Geometry check sheet. Reference: the model listing, model coordinates, mm. A direction names the side the tool comes from. Coordinates: 2 decimals unless noted, no trailing zeros. Order: outer loops, then holes, each group sorted by start corner. A loop starts at its lowest first (then second) coordinate and runs counter-clockwise, first axis right, second up. Notation, with made-up numbers: M 9.25,49.5 L 49.25,49.5 A8 ccw 49.25,58.5 Z; hole C 50.25,87.25 d8. An arc over 180 degrees is marked long. One line per item, written item: value. Start each with the question number.
1) Draft check along Z on faces 5 (the flat face through (-23, 0, 10)), 6 (the flat face through (22.47, 37.89, 16.47)), 7 (the flat face through (21.933, 37.891, 13.222)), 8 (the cylindrical face through (-0.323, -13.902, -15.247)). Enter one of: pulls with the +Z half, pulls with the -Z half, needs draft (parallel to the pull), parting line crosses it, or undercut.
2) Sectioned sample at B-B, the plane x = 0. Enter the section's corners in (y, z).
3) Sectioned sample at D-D, the plane y = 29.5. Enter the section's corners in (x, z), then the cut area to 3 significant figures.
4) Thickness scan on L1, parallel to X at y = 32.5, z = 0; L2, parallel to Y at x = -13.5, z = 24.5; L3, parallel to Y at x = -13, z = -30. Record the ranges inside material, lowest first. Write a range as from..to.
5) Go/stop test with flat-tipped pins: P1, Ø2, axis at x = 6.5, y = 30, coming from the -Z side; P2, Ø1.5, axis at y = 9.5, z = -1, coming from the -X side; P3, Ø3, axis at x = 25, y = 24.5, coming from the -Z side; P4, Ø1, axis at y = -13.5, z = 17, coming from the -X side. Record where each tip stops, or that it passes through.
6) Sectioned sample at A-A, the plane y = 37. Enter the section's corners in (x, z).
7) Access from +Z, -Z, +X, -X, +Y, -Y to the whole of each face (thin tool, end or side, straight path). Record for faces 1 (the flat face through (-23.08, 37.891, 15.624)), 2 (the flat face through (0, -15, 0.903)), 3 (the flat face through (0, 31.3, -28)), 4 (the flat face through (0, -7, 0)).
8) Sectioned sample at C-C, the plane y = -6. Enter the section's corners in (x, z).
```python
from build123d import *

# Parameters (mm, degrees)
SKETCH1_R           = 34
BOSS_EXTRUDE1_DEPTH = 44.3
SKETCH2_R           = 30
CUT_EXTRUDE1_DEPTH  = 37
SKETCH3_R           = 19.5
BOSS_EXTRUDE2_DEPTH = 7
SKETCH4_R           = 15.25
BOSS_EXTRUDE3_DEPTH = 16
FILLET1_R           = 5
BOSS_EXTRUDE4_DEPTH = 13
SKETCH7_W           = 66.193685288
SKETCH7_H           = 1.806726502
CUT_EXTRUDE2_DEPTH  = 16
FILLET2_R           = 2


with BuildPart() as part:
    # Sketch1 → Boss-Extrude1 (new body)
    with BuildSketch(Plane(origin=(0, 0, 0), x_dir=(1, 0, 0), z_dir=(0, 1, 0))):
        with Locations(Location((0, 0, 0), (0, 0, 270))):
            Circle(SKETCH1_R)
    extrude(amount=BOSS_EXTRUDE1_DEPTH)

    # Sketch2 → Cut-Extrude1 (cut)
    with BuildSketch(Plane(origin=(0, 44.3, 0), x_dir=(1, 0, 0), z_dir=(0, 1, 0))):
        with Locations(Location((0, 0, 0), (0, 0, 270))):
            Circle(SKETCH2_R)
    extrude(amount=-CUT_EXTRUDE1_DEPTH, mode=Mode.SUBTRACT)

    # Sketch3 → Boss-Extrude2 (add)
    with BuildSketch(Plane.XZ):
        with Locations(Location((0, 0, 0), (0, 0, 270))):
            Circle(SKETCH3_R)
    extrude(amount=BOSS_EXTRUDE2_DEPTH)

    # Sketch4 → Boss-Extrude3 (add)
    with BuildSketch(Plane.XZ.offset(7)):
        with Locations(Location((0, 0, 0), (0, 0, 270))):
            Circle(SKETCH4_R)
    extrude(amount=BOSS_EXTRUDE3_DEPTH)

    # Fillet1
    fillet1_edges = [part.edges().sort_by_distance(p)[0] for p in [
        (0, 0, 19.5),
    ]]
    fillet(fillet1_edges, radius=FILLET1_R)

    # Sketch5 → Boss-Extrude4 (add)
    with BuildSketch(Plane(origin=(0, 44.3, 0), x_dir=(1, 0, 0), z_dir=(0, 1, 0))):
        with BuildLine():
            Line((-1.990534123, 29.933890056), (-1.990534123, 25.605317076))
            Line((-1.990534123, 25.605317076), (3.030233114, 25.605317076))
            Line((3.030233114, 25.605317076), (3.030233114, 29.846569104))
            ThreePointArc((3.030233114, 29.846569104), (0.521679725, 29.995463828), (-1.990534123, 29.933890056))
        make_face()
        with BuildLine():
            Line((26.918776284, -13.243091911), (23.170122121, -11.07880542))
            Line((23.170122121, -11.07880542), (20.659738503, -15.426917394))
            Line((20.659738503, -15.426917394), (24.332770503, -17.547543408))
            ThreePointArc((24.332770503, -17.547543408), (25.715993811, -15.449519808), (26.918776284, -13.243091911))
        make_face()
        with BuildLine():
            Line((-24.928242161, -16.690798146), (-21.179587998, -14.526511655))
            Line((-21.179587998, -14.526511655), (-23.689971616, -10.178399682))
            Line((-23.689971616, -10.178399682), (-27.363003617, -12.299025696))
            ThreePointArc((-27.363003617, -12.299025696), (-26.237673536, -14.54594402), (-24.928242161, -16.690798146))
        make_face()
    extrude(amount=-BOSS_EXTRUDE4_DEPTH)

    # Sketch7 → Cut-Extrude2 (cut)
    with BuildSketch(Plane.XZ.offset(23)):
        Rectangle(SKETCH7_W, SKETCH7_H)
    extrude(amount=-CUT_EXTRUDE2_DEPTH, mode=Mode.SUBTRACT)

    # Fillet2
    fillet2_edges = [part.edges().sort_by_distance(p)[0] for p in [
        (0, -23, 15.25),
        (0, -23, -15.25),
    ]]
    fillet(fillet2_edges, radius=FILLET2_R)


solid = part.part
```
Final values:
1. face 5: needs draft
1. face 6: undercut
1. face 7: undercut
1. face 8: pulls with the -Z half
2. outline: M -23,-13.25 A2 ccw -21,-15.25 L -7,-15.25 L -7,-19.5 L -5,-19.5 A5 cw 0,-24.5 L 0,-34 L 44.3,-34 L 44.3,-25.61 L 31.3,-25.61 L 31.3,-30 L 7.3,-30 L 7.3,30 L 44.3,30 L 44.3,34 L 0,34 L 0,24.5 A5 cw -5,19.5 L -7,19.5 L -7,15.25 L -21,15.25 A2 ccw -23,13.25 L -23,0.9 L -7,0.9 L -7,-0.9 L -23,-0.9 Z
3. outline: C 0,0 d68; hole C 0,0 d60
3. area: 804 mm^2
4. L1: x = -34..-30, 30..34
4. L2: y = 0..7.3
4. L3: y = 0..44.3
5. P1: stops at z = -33.55
5. P2: stops at x = -34
5. P3: stops at z = -24.57
5. P4: passes through
6. outline: C 0,0 d68; hole M -27.36,12.3 A30 ccw -1.99,-29.93 L -1.99,-25.61 L 3.03,-25.61 L 3.03,-29.85 A30 ccw 26.92,13.24 L 23.17,11.08 L 20.66,15.43 L 24.33,17.55 A30 ccw -24.93,16.69 L -21.18,14.53 L -23.69,10.18 Z
7. face 1: +Y
7. face 2: +X, -X, -Y
7. face 3: none
7. face 4: -Y
8. outline: C 0,0 d39
